```python
from build123d import *

# Parameters (mm, degrees)
MODEL_R                 = 1.75
MODEL_W                 = 3
MODEL_H                 = 3
MODEL_W_2               = 3.000000001
SALIENTE_EXTRUIR1_DEPTH = 3


with BuildPart() as part:
    # Model → Saliente-Extruir1 (new body)
    with BuildSketch(Plane.XY):
        with BuildLine():
            Line((10.922877124, 294.963401588), (64.922877125, 294.963401588))
            ThreePointArc((64.922877125, 294.963401588), (68.10485764, 293.645382103), (69.422877125, 290.463401588))
            Line((69.422877125, 290.463401588), (69.422877125, 254.463401588))
            ThreePointArc((69.422877125, 254.463401588), (68.10485764, 251.281421073), (64.922877125, 249.963401588))
            Line((64.922877125, 249.963401588), (10.922877124, 249.963401588))
            ThreePointArc((10.922877124, 249.963401588), (7.740896609, 251.281421073), (6.422877125, 254.463401588))
            Line((6.422877125, 254.463401588), (6.422877125, 290.463401588))
            ThreePointArc((6.422877125, 290.463401588), (7.740896609, 293.645382103), (10.922877124, 294.963401588))
        make_face()
        with Locations((64.922877125, 284.463401588)):
            Circle(MODEL_R, mode=Mode.SUBTRACT)
        with Locations((34.922877124, 284.463401588)):
            Circle(MODEL_R, mode=Mode.SUBTRACT)
        with Locations((64.922877125, 260.463401588)):
            Circle(MODEL_R, mode=Mode.SUBTRACT)
        with Locations((34.922877124, 260.463401588)):
            Circle(MODEL_R, mode=Mode.SUBTRACT)
        with Locations((40.922877124, 284.463401588)):
            Circle(MODEL_R, mode=Mode.SUBTRACT)
        with Locations((10.922877124, 284.463401588)):
            Circle(MODEL_R, mode=Mode.SUBTRACT)
        with Locations((40.922877124, 260.463401588)):
            Circle(MODEL_R, mode=Mode.SUBTRACT)
        with Locations((10.922877124, 260.463401588)):
            Circle(MODEL_R, mode=Mode.SUBTRACT)
        with Locations((10.922877124, 290.463401588)):
            Rectangle(MODEL_W, MODEL_H, mode=Mode.SUBTRACT)
        with Locations((19.922877124, 290.463401588)):
            Rectangle(MODEL_W, MODEL_H, mode=Mode.SUBTRACT)
        with Locations((28.922877124, 290.463401588)):
            Rectangle(MODEL_W, MODEL_H, mode=Mode.SUBTRACT)
        with Locations((55.922877124, 290.463401588)):
            Rectangle(MODEL_W, MODEL_H, mode=Mode.SUBTRACT)
        with Locations((64.922877125, 290.463401588)):
            Rectangle(MODEL_W_2, MODEL_H, mode=Mode.SUBTRACT)
        with Locations((10.922877124, 254.463401588)):
            Rectangle(MODEL_W, MODEL_H, mode=Mode.SUBTRACT)
        with Locations((19.922877124, 254.463401588)):
            Rectangle(MODEL_W, MODEL_H, mode=Mode.SUBTRACT)
        with Locations((28.922877124, 254.463401588)):
            Rectangle(MODEL_W, MODEL_H, mode=Mode.SUBTRACT)
        with Locations((55.922877124, 254.463401588)):
            Rectangle(MODEL_W, MODEL_H, mode=Mode.SUBTRACT)
        with Locations((64.922877125, 254.463401588)):
            Rectangle(MODEL_W_2, MODEL_H, mode=Mode.SUBTRACT)
        with Locations((19.922877124, 263.463401588)):
            Rectangle(MODEL_W, MODEL_H, mode=Mode.SUBTRACT)
        with Locations((28.922877124, 263.463401588)):
            Rectangle(MODEL_W, MODEL_H, mode=Mode.SUBTRACT)
        with Locations((55.922877124, 263.463401588)):
            Rectangle(MODEL_W, MODEL_H, mode=Mode.SUBTRACT)
        with Locations((37.922877124, 290.463401588)):
            Rectangle(MODEL_W, MODEL_H, mode=Mode.SUBTRACT)
        with Locations((46.922877124, 290.463401588)):
            Rectangle(MODEL_W, MODEL_H, mode=Mode.SUBTRACT)
        with Locations((37.922877124, 254.463401588)):
            Rectangle(MODEL_W, MODEL_H, mode=Mode.SUBTRACT)
        with Locations((46.922877124, 254.463401588)):
            Rectangle(MODEL_W, MODEL_H, mode=Mode.SUBTRACT)
        with Locations((46.922877124, 263.463401588)):
            Rectangle(MODEL_W, MODEL_H, mode=Mode.SUBTRACT)
        with Locations((10.922877124, 272.463401588)):
            Rectangle(MODEL_W, MODEL_H, mode=Mode.SUBTRACT)
        with Locations((19.922877124, 272.463401588)):
            Rectangle(MODEL_W, MODEL_H, mode=Mode.SUBTRACT)
        with Locations((28.922877124, 272.463401588)):
            Rectangle(MODEL_W, MODEL_H, mode=Mode.SUBTRACT)
        with Locations((55.922877124, 272.463401588)):
            Rectangle(MODEL_W, MODEL_H, mode=Mode.SUBTRACT)
        with Locations((64.922877125, 272.463401588)):
            Rectangle(MODEL_W_2, MODEL_H, mode=Mode.SUBTRACT)
        with Locations((19.922877124, 281.463401588)):
            Rectangle(MODEL_W, MODEL_H, mode=Mode.SUBTRACT)
        with Locations((28.922877124, 281.463401588)):
            Rectangle(MODEL_W, MODEL_H, mode=Mode.SUBTRACT)
        with Locations((55.922877124, 281.463401588)):
            Rectangle(MODEL_W, MODEL_H, mode=Mode.SUBTRACT)
        with Locations((37.922877124, 272.463401588)):
            Rectangle(MODEL_W, MODEL_H, mode=Mode.SUBTRACT)
        with Locations((46.922877124, 272.463401588)):
            Rectangle(MODEL_W, MODEL_H, mode=Mode.SUBTRACT)
        with Locations((46.922877124, 281.463401588)):
            Rectangle(MODEL_W, MODEL_H, mode=Mode.SUBTRACT)
    extrude(amount=SALIENTE_EXTRUIR1_DEPTH)


solid = part.part
```
Part model, mm, in its own coordinate system. A direction names the side the tool comes from. Round coordinates to 2 decimals unless told otherwise and drop trailing zeros. Write each loop counter-clockwise with the first axis right and the second up, starting at its lowest first coordinate (ties: lowest second). Pieces come first, ordered by that corner, then holes. Notation, with made-up numbers: M -1,34 L 57,34 A22 ccw 57,65 Z; hole C -27,78.5 d6. An arc over 180 degrees is marked long. Answer as CSV lines item,"result". Start each with the question number.
1) Mould opens along X. For faces 3 (the face through (29, 261.963, 1)), 4 (the face through (38, 249.963, 1)), 5 (the face through (7.776, 251.247, 1.479)) say: +X half, -X half, draft (parallel to the pull), parting line (faces both ways), or undercut.
2) Drop a flat-ended pin along its axis: pin 1 (3 mm diameter, centred on x = 40.92, y = 284.46, fed in from -Z). Give the stop position or say it passes through.
3) Band-saw the part on A-A (x = 42). List the corners of the cut face in (y, z), then the cut area to 3 significant figures.
4) Drill centre lines: L1, parallel to Y at x = 39, z = 0.55; L2, parallel to Y at x = 41, z = 2.6; L3, parallel to Y at x = 55.5, z = 2.25. Where is each one in solid material? Low to high.
5) Band-saw the part on B-B (z = 1.6). Count the separate pieces of the cut face and the enclosed holes in it, then the cut area to 3 significant figures.
6) Which spindle directions (+Z, -Z, +X, -X, +Y, -Y) get a long thin tool onto all of the face, cutting with end or side? Do faces 1 (the face through (7.706, 293.61, 1.479)), 2 (the face through (9.423, 272, 1)). Say none if no direction does.
Worked out:
1,face 3,"undercut"
1,face 4,"draft"
1,face 5,"-X half"
2,pin 1,"through"
3,outline,"M 249.96,0 L 259.08,0 L 259.08,3 L 249.96,3 Z; M 261.84,0 L 283.08,0 L 283.08,3 L 261.84,3 Z; M 285.84,0 L 294.96,0 L 294.96,3 L 285.84,3 Z"
3,area,"118 mm²"
4,L1,"249.96 to 252.96, 255.96 to 270.96, 273.96 to 288.96, 291.96 to 294.96"
4,L2,"249.96 to 258.72, 262.21 to 282.72, 286.21 to 294.96"
4,L3,"249.96 to 252.96, 255.96 to 261.96, 264.96 to 270.96, 273.96 to 279.96, 282.96 to 288.96, 291.96 to 294.96"
5,separate pieces,"1"
5,enclosed holes,"37"
5,area,"2,480 mm²"
6,face 1,"+Z, -Z, -X, +Y"
6,face 2,"+Z, -Z"
